from build123d import *

# Parameters (mm, degrees)
REVOLVE1_ANGLE     = 180
SKETCH3_W          = 24.5
SKETCH3_H          = 53.5
CUT_EXTRUDE1_DEPTH = 7
SKETCH4_W          = 9.5
SKETCH4_H          = 7
CUT_EXTRUDE2_DEPTH = 2.5
SKETCH5_W          = 6
SKETCH5_H          = 10
CUT_EXTRUDE3_DEPTH = 2.5


with BuildPart() as part:
    # Sketch2 → Revolve1 (revolve)
    with BuildSketch(Plane(origin=(0, 0, 0), x_dir=(1, 0, 0), z_dir=(0, 1, 0))):
        Polygon((0, 0), (-15, 0), (-15, 64), (-9, 64), (-9, 144), (-3, 165), (0, 165), align=None)
    revolve(axis=Axis((0, 0, -165), (0, 0, 1)), revolution_arc=REVOLVE1_ANGLE)

    # Sketch3 → Cut-Extrude1 (cut)
    with BuildSketch(Plane(origin=(0, 0, 0), x_dir=(1, 0, 0), z_dir=(0, 1, 0))):
        with Locations((0, 32.132467542)):
            Rectangle(SKETCH3_W, SKETCH3_H)
    extrude(amount=-CUT_EXTRUDE1_DEPTH, mode=Mode.SUBTRACT)

    # Sketch4 → Cut-Extrude2 (cut)
    with BuildSketch(Plane(origin=(0, 0, 0), x_dir=(1, 0, 0), z_dir=(0, 1, 0))):
        with Locations((0, 62.382467542)):
            Rectangle(SKETCH4_W, SKETCH4_H)
    extrude(amount=-CUT_EXTRUDE2_DEPTH, mode=Mode.SUBTRACT)

    # Sketch5 → Cut-Extrude3 (cut)
    with BuildSketch(Plane(origin=(0, 0, 0), x_dir=(1, 0, 0), z_dir=(0, 1, 0))):
        with Locations((0, 100.5)):
            Rectangle(SKETCH5_W, SKETCH5_H)
    extrude(amount=-CUT_EXTRUDE3_DEPTH, mode=Mode.SUBTRACT)


solid = part.part
Build history of the part. All positions in model axes, mm. A direction names the side the tool comes from. Give positions to 0.01 mm unless a question says otherwise; leave off trailing zeros. Order: outer loops, then holes, each group sorted by start corner. A loop starts at its lowest first (then second) coordinate and runs counter-clockwise, first axis right, second up. Notation, with made-up numbers: M -23.5,-32 L 10.5,-32 A10 cw 10.5,-18 Z; hole C 61,7.5 d5. An arc over 180 degrees is marked long. Use one line per item in the form item = value.
1) Saw through at A-A (x = 0). Give the cut face in (y, z).
Calculated:
outline = M -15,-64 L -9,-64 L -9,-144 L -3,-165 L 0,-165 L 0,-105.5 L -2.5,-105.5 L -2.5,-95.5 L 0,-95.5 L 0,-65.88 L -2.5,-65.88 L -2.5,-58.88 L -7,-58.88 L -7,-5.38 L 0,-5.38 L 0,0 L -15,0 Z
2) Probe probe 1 along Z at (x, y) = (-2, -1); probe 2 along Z at (x, y) = (11.25, -5.5); probe 3 along X at (y, z) = (-4, -45.5). List the from-to ranges inside material, lowest first.
Calculated:
probe_1 = -165 to -105.5, -95.5 to -65.88, -5.38 to 0
probe_2 = -64 to -58.88, -5.38 to 0
probe_3 = -14.46 to -12.25, 12.25 to 14.46
3) Tool access for faces 1 (the face through (-12.25, -3, -32)), 2 (the face through (0, -1, -165)), 3 (the face through (0, -9, -105)): list every direction of +Z, -Z, +X, -X, +Y, -Y with a clear straight run to the whole face (end or side of a thin tool).
Calculated:
face_1 = +Y
face_2 = -Z, +X, -X, +Y, -Y
face_3 = -Z, -Y
4) Saw through at C-C (z = -81). Give the cut face in (x, y).
Calculated:
outline = M -9,0 A9 ccw 9,0 Z
5) Saw through at B-B (z = -41.5). Give the cut face in (x, y), plus the area to 3 significant figures.
Calculated:
outline = M -15,0 A15 ccw 15,0 L 12.25,0 L 12.25,-7 L -12.25,-7 L -12.25,0 Z
area = 182 mm2
6) Drop flat-ended pins along their axis: pin 1 (3.5 mm diameter, centred on x = -2, z = -62.5, fed in from +Y); pin 2 (3.5 mm diameter, centred on y = -3, z = -42.5, fed in from +X); pin 3 (2 mm diameter, centred on y = -1.5, z = -62.5, fed in from +X). Give the stop position or say it passes through.
Calculated:
pin_1 = -2.5
pin_2 = 14.95
pin_3 = 14.99
7) Two-plate mould, pull along Z, no slides. Class faces 4 (the face through (0, -2.5, -101)), 5 (the face through (0, -6, 0)), 6 (the face through (-0.131, -5.957, -154.647)): released by +Z, released by -Z, zero draft, split by the parting line, or undercut.
Calculated:
face_4 = undercut
face_5 = released by +Z
face_6 = released by -Z
